from build123d import *

# Parameters (mm, degrees)
CROQUIS1_R              = 1.05
SALIENTE_EXTRUIR1_DEPTH = 2


with BuildPart() as part:
    # Croquis1 → Saliente-Extruir1 (new body)
    with BuildSketch(Plane(origin=(0, 0, 0), x_dir=(1, 0, 0), z_dir=(0, 1, 0))):
        with BuildLine():
            Line((-11.2, 0), (-11.2, 12))
            Line((-11.2, 12), (11.2, 12))
            Line((11.2, 12), (11.2, 0))
            Line((11.2, 0), (12.25, 0))
            Line((12.25, 0), (12.25, -3))
            Line((12.25, -3), (15.75, -3))
            Line((15.75, -3), (15.75, 0))
            Line((15.75, 0), (16.8, 0))
            Line((16.8, 0), (16.8, 9))
            ThreePointArc((16.8, 9), (15.335533906, 12.535533906), (11.8, 14))
            Line((11.8, 14), (-11.8, 14))
            ThreePointArc((-11.8, 14), (-15.335533906, 12.535533906), (-16.8, 9))
            Line((-16.8, 9), (-16.8, 0))
            Line((-16.8, 0), (-15.75, 0))
            Line((-15.75, 0), (-15.75, -3))
            Line((-15.75, -3), (-12.25, -3))
            Line((-12.25, -3), (-12.25, 0))
            Line((-12.25, 0), (-11.2, 0))
        make_face()
        with Locations(Location((-14, 6, 0), (0, 0, 270))):
            Circle(CROQUIS1_R, mode=Mode.SUBTRACT)
        with Locations(Location((14, 6, 0), (0, 0, 270))):
            Circle(CROQUIS1_R, mode=Mode.SUBTRACT)
    extrude(amount=SALIENTE_EXTRUIR1_DEPTH)


solid = part.part
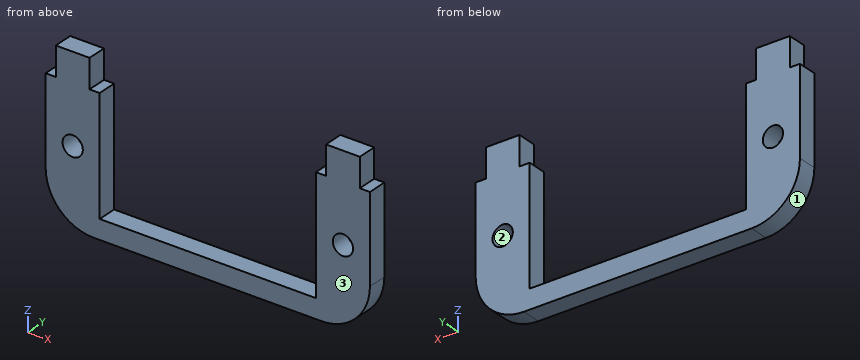
Source: CAD feature listing. Evaluate the final solid. Frame: model axes, mm. Face numbers are marked on the shaded views. Round coordinates to 2 decimals unless told otherwise and drop trailing zeros. Loops run counter-clockwise (first coordinate to the right, second up) from the corner with the lowest first, then second, coordinate; pieces in that order, holes last. Notation, with made-up numbers: (75, 62) - (102, 62) arc R20 ccw to (102, 92) - close; hole circle Ø9 at (-19.5, 32.5). An arc over 180 degrees is marked (long way). Write item = value, one per line. Start each with the question number.
(1) Section query A-A, the plane z = -6. Output: boundary loops of the cut face in (x, y), plus the area to 3 significant figures.
(2) Section query D-D, the plane z = -3. Output: boundary loops of the cut face in (x, y).
(3) Section query C-C, the plane x = 14. Output: boundary loops of the cut face in (y, z), plus the area to 3 significant figures.
(4) Pull-direction query (Z, two-part tool) for the marked faces 1, 2 and 3; classes: +Z half, -Z half, draft (parallel to the pull), parting line (faces both ways), or undercut.
(5) Ray query, line 1 along X through (y, z) = (1.1, -6); line 2 along X through (y, z) = (0.2, 2.75); line 3 along Z through (x, y) = (-8, 1.1). Return the intervals inside material, ascending. Write a range as from..to.
(6) Section query B-B, the plane y = 0.8. Output: boundary loops of the cut face in (x, z), plus the area to 3 significant figures.
(7) Pin query (flat end, axial travel): pin 1 (0.6 mm diameter, centred on y = 0.5, z = 1, fed in from -X); pin 2 (1.2 mm diameter, centred on x = 11.5, y = 1, fed in from +Z); pin 3 (0.6 mm diameter, centred on x = 0, y = 1, fed in from +Z). Return the tip coordinate at first contact, or that it passes through.
Conclusion:
q1.outline = (-16.8, 0) - (-15.05, 0) - (-15.05, 2) - (-16.8, 2) - close; (-12.95, 0) - (-11.2, 0) - (-11.2, 2) - (-12.95, 2) - close; (11.2, 0) - (12.95, 0) - (12.95, 2) - (11.2, 2) - close; (15.05, 0) - (16.8, 0) - (16.8, 2) - (15.05, 2) - close
q1.area = 14.0 mm2
q2.outline = (-16.8, 0) - (-11.2, 0) - (-11.2, 2) - (-16.8, 2) - close; (11.2, 0) - (16.8, 0) - (16.8, 2) - (11.2, 2) - close
q3.outline = (0, -13.49) - (2, -13.49) - (2, -7.05) - (0, -7.05) - close; (0, -4.95) - (2, -4.95) - (2, 3) - (0, 3) - close
q3.area = 28.8 mm2
q4.face_1 = -Z half
q4.face_2 = undercut
q4.face_3 = draft
q5.line_1 = -16.8..-15.05, -12.95..-11.2, 11.2..12.95, 15.05..16.8
q5.line_2 = -15.75..-12.25, 12.25..15.75
q5.line_3 = -14..-12
q6.outline = (-16.8, -9) arc R5 ccw to (-11.8, -14) - (11.8, -14) arc R5 ccw to (16.8, -9) - (16.8, 0) - (15.75, 0) - (15.75, 3) - (12.25, 3) - (12.25, 0) - (11.2, 0) - (11.2, -12) - (-11.2, -12) - (-11.2, 0) - (-12.25, 0) - (-12.25, 3) - (-15.75, 3) - (-15.75, 0) - (-16.8, 0) - close; hole circle Ø2.1 at (-14, -6); hole circle Ø2.1 at (14, -6)
q6.area = 205 mm2
q7.pin_1 = -15.75
q7.pin_2 = 0
q7.pin_3 = -12
